from build123d import *

# Parameters (mm, degrees)
SKETCH1_W           = 65
SKETCH1_H           = 95
BOSS_EXTRUDE1_DEPTH = 45
SHELL4_T            = 4
SKETCH3_W           = 65
SKETCH3_H           = 5
BOSS_EXTRUDE3_DEPTH = 15
SKETCH4_R           = 5
SKETCH4_R_2         = 5.5
CUT_EXTRUDE1_DEPTH  = 5
FILLET1_R           = 4
FILLET2_R           = 2


with BuildPart() as part:
    # Sketch1 → Boss-Extrude1 (new body)
    with BuildSketch(Plane(origin=(0, 0, 0), x_dir=(1, 0, 0), z_dir=(0, 1, 0))):
        Rectangle(SKETCH1_W, SKETCH1_H)
    extrude(amount=BOSS_EXTRUDE1_DEPTH)

    # Shell4
    shell4_openings = [part.faces().sort_by_distance(p)[0] for p in [
        (0, 45, 0),
    ]]
    offset(amount=SHELL4_T, openings=shell4_openings, kind=Kind.INTERSECTION)

    # Sketch3 → Boss-Extrude3 (add)
    with BuildSketch(Plane(origin=(0, 0, 0), x_dir=(1, 0, 0), z_dir=(0, 1, 0))):
        with Locations((0, 13)):
            Rectangle(SKETCH3_W, SKETCH3_H)
    extrude(amount=BOSS_EXTRUDE3_DEPTH)

    # Sketch4 → Cut-Extrude1 (cut)
    with BuildSketch(Plane(origin=(-32.5, 0, 0), x_dir=(0, 0, -1), z_dir=(1, 0, 0))):
        with Locations((9.5, 30)):
            Circle(SKETCH4_R)
        with Locations((-9.5, 30)):
            Circle(SKETCH4_R_2)
    extrude(amount=-CUT_EXTRUDE1_DEPTH, mode=Mode.SUBTRACT)

    # Fillet1
    fillet1_edges = [part.edges().sort_by_distance(p)[0] for p in [
        (0, -4, 51.5),
        (-36.5, -4, 0),
        (0, -4, -51.5),
        (36.5, -4, 0),
        (36.5, 20.5, 51.5),
        (-36.5, 20.5, 51.5),
        (-36.5, 20.5, -51.5),
        (36.5, 20.5, -51.5),
    ]]
    fillet(fillet1_edges, radius=FILLET1_R)

    # Fillet2
    fillet2_edges = [part.edges().sort_by_distance(p)[0] for p in [
        (0, 15, -10.5),
        (0, 15, -15.5),
    ]]
    fillet(fillet2_edges, radius=FILLET2_R)


solid = part.part
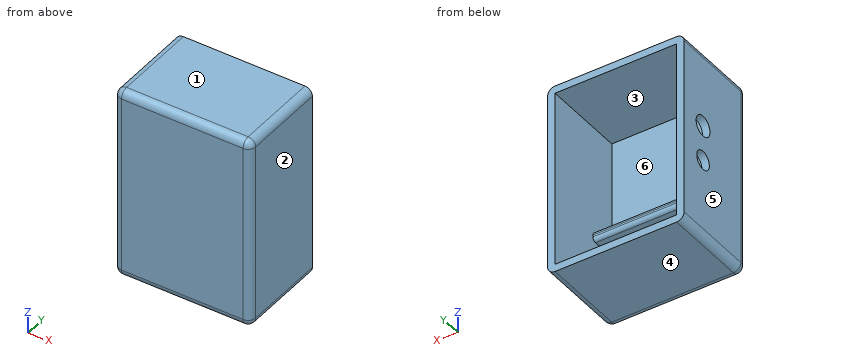
Geometry check sheet. Reference: the model listing, model coordinates, mm. Face numbers are marked on the shaded views. A direction names the side the tool comes from. Round coordinates to 2 decimals unless told otherwise and drop trailing zeros. Write each loop counter-clockwise with the first axis right and the second up, starting at its lowest first coordinate (ties: lowest second). Pieces come first, ordered by that corner, then holes. Notation, with made-up numbers: (-35.75, 65) - (-31.75, 65) arc R18 ccw to (-31.75, 90) - close; hole circle Ø9 at (68.5, 29.25). An arc over 180 degrees is marked (long way). One line per item, written item: value.
1. Cross-section at D-D on x = 17. Record the boundary of the cut face in (y, z), and give its area (3 significant figures).
The answers:
outline: (-4, -47.5) arc R4 ccw to (0, -51.5) - (45, -51.5) - (45, -47.5) - (0, -47.5) - (0, -15.5) - (13, -15.5) arc R2 ccw to (15, -13.5) - (15, -12.5) arc R2 ccw to (13, -10.5) - (0, -10.5) - (0, 47.5) - (45, 47.5) - (45, 51.5) - (0, 51.5) arc R4 ccw to (-4, 47.5) - close
area: 838 mm^2
2. Cross-section at C-C on y = 6.5. Record the boundary of the cut face in (x, z).
The answers:
outline: (-36.5, -47.5) arc R4 ccw to (-32.5, -51.5) - (32.5, -51.5) arc R4 ccw to (36.5, -47.5) - (36.5, 47.5) arc R4 ccw to (32.5, 51.5) - (-32.5, 51.5) arc R4 ccw to (-36.5, 47.5) - close; hole (-32.5, -47.5) - (32.5, -47.5) - (32.5, -15.5) - (-32.5, -15.5) - close; hole (-32.5, -10.5) - (32.5, -10.5) - (32.5, 47.5) - (-32.5, 47.5) - close
3. Mould release check, pull along Z, two halves, no side actions. Record for the marked faces 1, 2, 3 and 4: released by +Z, released by -Z, zero draft, split by the parting line, or undercut.
The answers:
face 1: released by +Z
face 2: zero draft
face 3: undercut
face 4: released by -Z
4. Cross-section at A-A on z = 9.5. Record the boundary of the cut face in (x, y), and give its area (3 significant figures).
The answers:
outline: (-36.5, 0) arc R4 ccw to (-32.5, -4) - (32.5, -4) arc R4 ccw to (36.5, 0) - (36.5, 45) - (32.5, 45) - (32.5, 0) - (-32.5, 0) - (-32.5, 24.5) - (-36.5, 24.5) - close; (-36.5, 35.5) - (-32.5, 35.5) - (-32.5, 45) - (-36.5, 45) - close
area: 601 mm^2
5. Set-up check for the marked faces 5 and 6: record each of +Z, -Z, +X, -X, +Y, -Y from which the full face is reachable in a straight line by a thin tool's end or side.
The answers:
face 5: +Z, -Z, -X, +Y, -Y
face 6: +Y
6. Depth check by flat-ended pin: pin 1 Ø8 at (y, z) = (30, -9.5) entering from -X. Enter the tip coordinate at first touch or a pass-through.
The answers:
pin 1: stops at x = 32.5
7. Scan lines: L1, parallel to Z at x = -3, y = 6; L2, parallel to X at y = 7, z = -42.5; L3, parallel to Z at x = 3.5, y = 37. Record each from-to range of solid material in increasing order.
The answers:
L1: z = -51.5 to -47.5, -15.5 to -10.5, 47.5 to 51.5
L2: x = -36.5 to -32.5, 32.5 to 36.5
L3: z = -51.5 to -47.5, 47.5 to 51.5
8. Cross-section at B-B on y = 18. Record the boundary of the cut face in (x, z).
The answers:
outline: (-36.5, -47.5) arc R4 ccw to (-32.5, -51.5) - (32.5, -51.5) arc R4 ccw to (36.5, -47.5) - (36.5, 47.5) arc R4 ccw to (32.5, 51.5) - (-32.5, 51.5) arc R4 ccw to (-36.5, 47.5) - close; hole (-32.5, -47.5) - (32.5, -47.5) - (32.5, 47.5) - (-32.5, 47.5) - close
